The figure shows three views and two pictorial views of one solid part (mm, origin at its lowest corner). Answer the questions. A direction names the side the tool comes from. Coordinates: 2 decimals unless noted, no trailing zeros. Write each loop counter-clockwise with the first axis right and the second up, starting at its lowest first coordinate (ties: lowest second). Pieces come first, ordered by that corner, then holes.
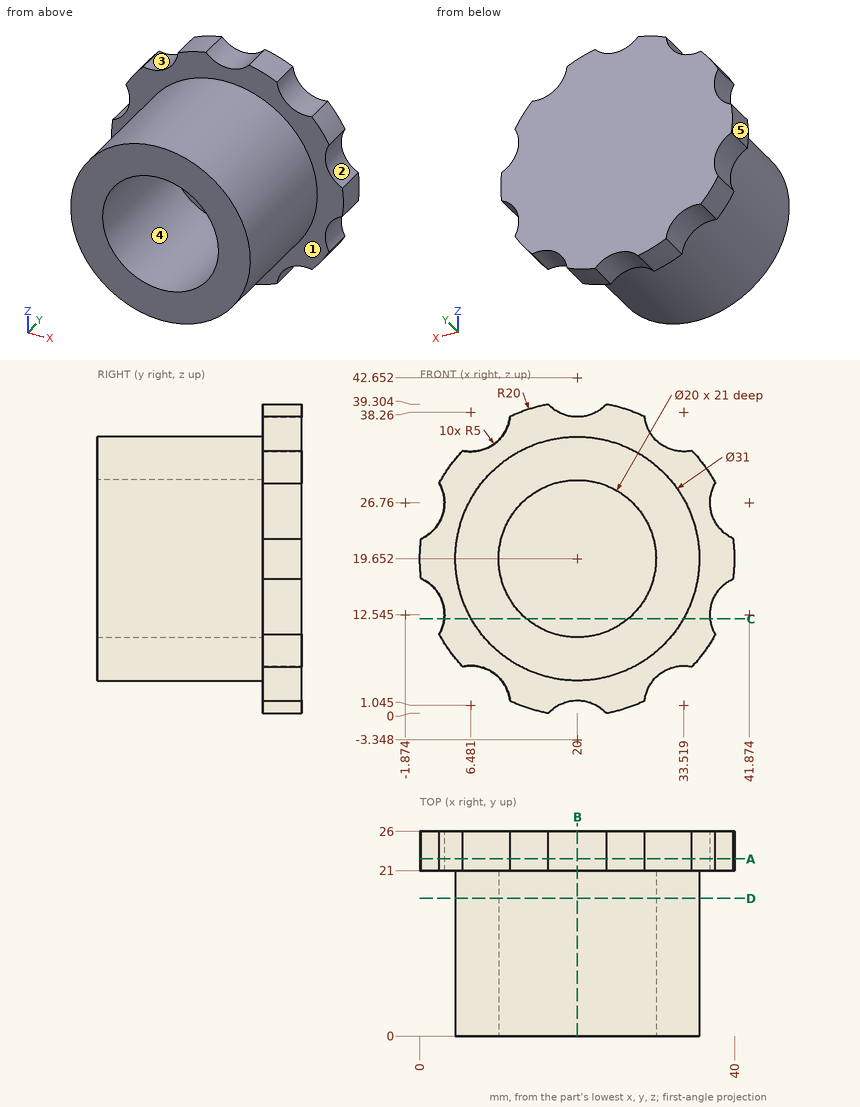
Q1. Find the intervals of material crossed by probe 1 along X at (y, z) = (3, 20); probe 2 along X at (y, z) = (20, 16) (1 decimal); probe 3 along Z at (x, y) = (11, 20.75) (1 decimal), in increasing order.
Answers below:
probe 1: x = 4.5 to 10.01, 29.99 to 35.5
probe 2: x = 4.9 to 10.7, 29.3 to 35.1
probe 3: z = 7 to 15.3, 24 to 32.3
Q2. Given pin 1 (22 mm diameter, centred on x = 17, z = 23, fed in from -Y); pin 2 (6 mm diameter, centred on x = 4, y = 3, fed in from -Z); pin 3 (12 mm diameter, centred on y = 8.5, z = 9, fed in from -X) (1 decimal); pin 4 (3 mm diameter, centred on y = 17.5, z = 16.5, fed in from -X), each flat-ended and moving along its own axis, determine where each tip first touches the part or whether it passes through.
Answers below:
pin 1: stops at y = 0
pin 2: stops at z = 11.21
pin 3: stops at x = 5.2
pin 4: stops at x = 4.59
Q3. Determine the mould class of the marked faces 1, 2 and 3 for opening direction Z: released by +Z, released by -Z, zero draft, split by the parting line, or undercut.
Answers below:
face 1: zero draft
face 2: undercut
face 3: released by +Z
Q4. The part is cut by section B-B, the plane x = 20. Write down the section's boundary in (y, z).
Answers below:
outline: (0, 4.15) - (21, 4.15) - (21, 1.65) - (26, 1.65) - (26, 37.65) - (21, 37.65) - (21, 35.15) - (0, 35.15) - (0, 29.65) - (21, 29.65) - (21, 9.65) - (0, 9.65) - close
Q5. The part is cut by section C-C, the plane z = 12. Write down the section's boundary in (x, y), then the cut area to 3 significant figures.
Answers below:
outline: (3.1, 21) - (6.52, 21) - (6.52, 0) - (13.56, 0) - (13.56, 21) - (26.44, 21) - (26.44, 0) - (33.48, 0) - (33.48, 21) - (36.9, 21) - (36.9, 26) - (3.1, 26) - close
area: 465 mm2
Q6. The part is cut by section D-D, the plane y = 17.5. Write down the section's boundary in (x, z).
Answers below:
outline: circle Ø31 at (20, 19.65); hole circle Ø20 at (20, 19.65)
Q7. Which of the six approach directions +Z, -Z, +X, -X, +Y, -Y give full straight-line access (tool end or side, diameter ignored) to the marked faces 4 and 5?
Answers below:
face 4: -Y
face 5: -X, +Y, -Y
Q8. The part is cut by section A-A, the plane y = 22.5. Write down the section's boundary in (x, z) (1 decimal), then the cut area to 3 significant figures.
Answers below:
outline: (0.2, 17.1) arc R5 cw to (2.5, 10) arc R20 ccw to (5.4, 5.9) arc R5 cw to (11.5, 1.6) arc R20 ccw to (16.3, 0) arc R5 cw to (23.7, 0) arc R20 ccw to (28.5, 1.6) arc R5 cw to (34.6, 5.9) arc R20 ccw to (37.5, 10) arc R5 cw to (39.8, 17.1) arc R20 ccw to (39.8, 22.2) arc R5 cw to (37.5, 29.3) arc R20 ccw to (34.6, 33.4) arc R5 cw to (28.5, 37.7) arc R20 ccw to (23.7, 39.3) arc R5 cw to (16.3, 39.3) arc R20 ccw to (11.5, 37.7) arc R5 cw to (5.4, 33.4) arc R20 ccw to (2.5, 29.3) arc R5 cw to (0.2, 22.2) arc R20 ccw to start
area: 1,150 mm2
